```python
from build123d import *

# Parameters (mm, degrees)
F0_R     = 7.5
F0_R_2   = 6.5
F1_DEPTH = 2.5
F0_R_3   = 4
F2_DEPTH = 2
F0_R_4   = 3
F3_DEPTH = 2.5


with BuildPart() as f1:
    # F0 (on Front) → F1 (new body, symmetric)
    with BuildSketch(Plane.XZ):
        Circle(F0_R)
        Circle(F0_R_2, mode=Mode.SUBTRACT)
    extrude(amount=F1_DEPTH, both=True)

    # F0 (on Front) → F2 (join, symmetric)
    with BuildSketch(Plane.XZ):
        Circle(F0_R_2)
        Circle(F0_R_3, mode=Mode.SUBTRACT)
    extrude(amount=F2_DEPTH, both=True)

    # F0 (on Front) → F3 (join, symmetric)
    with BuildSketch(Plane.XZ):
        Circle(F0_R_3)
        Circle(F0_R_4, mode=Mode.SUBTRACT)
    extrude(amount=F3_DEPTH, both=True)


solid = f1.part
```
The model under review builds one solid part; all positions refer to its coordinate system, in mm. A direction names the side the tool comes from. Round coordinates to 2 decimals unless told otherwise and drop trailing zeros. Loops run counter-clockwise (first coordinate to the right, second up) from the corner with the lowest first, then second, coordinate; pieces in that order, holes last. Notation, with made-up numbers: (-36.5, 19.5) - (-10.5, 19.5) arc R21 cw to (-10.5, 42.5) - close; hole circle Ø2 at (42, -0.75). An arc over 180 degrees is marked (long way). Write each question's results on one line, items separated by ' | '. Start each with the question number.
Q1. Take a section at B-B on x = 0. Give the boundary of the cut face in (y, z), plus the area to 3 significant figures.
Q2. Wall thickness on line 1 along Z through (x, y) = (0, 2.3); line 2 along Z through (x, y) = (0, -1.25); line 3 along Y through (x, z) = (-2, 4): over which ranges is each line inside the solid? List them lowest first. Write a range as [from, to].
Q3. Take a section at A-A on z = 0. Give the boundary of the cut face in (x, y), plus the area to 3 significant figures.
Q4. Take a section at D-D on x = -5.75. Give the boundary of the cut face in (y, z), plus the area to 3 significant figures.
Q5. Take a section at C-C on y = -0.8. Give the boundary of the cut face in (x, z), plus the area to 3 significant figures.
Q6. Draft analysis for pull direction Z (two halves, no side actions). For faces 1 (the cylindrical face through (-5.158, -2.246, -3.955)), 2 (the cylindrical face through (-7.493, -0.035, 0.33)), 3 (the flat face through (1, -2.5, 3)), state which applies: pulls with the +Z half, pulls with the -Z half, needs draft (parallel to the pull), parting line crosses it, or undercut.
Q7. Tool access review of faces 4 (the flat face through (1, 2.5, 3)), 5 (the cylindrical face through (-5.158, 2.254, -3.955)), 6 (the flat face through (3, -2, 3)): name each direction out of +Z, -Z, +X, -X, +Y, -Y from which nothing blocks a thin tool from reaching the whole face with its end or side.
Q8. Insertion check: P1, Ø1.5, axis at x = 2.5, y = 1, coming from the -Z side; P2, Ø3, axis at x = -5.5, y = 1.5, coming from the +Z side; P3, Ø1, axis at x = 6, y = 1, coming from the -Z side. Each pin has a flat end and moves straight along its axis. Give the tip position at first contact, or say it passes through.
Data:
1) outline: (-2.5, -7.5) - (2.5, -7.5) - (2.5, -6.5) - (2, -6.5) - (2, -4) - (2.5, -4) - (2.5, -3) - (-2.5, -3) - (-2.5, -4) - (-2, -4) - (-2, -6.5) - (-2.5, -6.5) - close; (-2.5, 3) - (2.5, 3) - (2.5, 4) - (2, 4) - (2, 6.5) - (2.5, 6.5) - (2.5, 7.5) - (-2.5, 7.5) - (-2.5, 6.5) - (-2, 6.5) - (-2, 4) - (-2.5, 4) - close | area: 40.0 mm²
2) line 1: z = [-7.5, -6.5], [-4, -3], [3, 4], [6.5, 7.5] | line 2: z = [-7.5, -3], [3, 7.5] | line 3: y = [-2, 2]
3) outline: (-7.5, -2.5) - (-6.5, -2.5) - (-6.5, -2) - (-4, -2) - (-4, -2.5) - (-3, -2.5) - (-3, 2.5) - (-4, 2.5) - (-4, 2) - (-6.5, 2) - (-6.5, 2.5) - (-7.5, 2.5) - close; (3, -2.5) - (4, -2.5) - (4, -2) - (6.5, -2) - (6.5, -2.5) - (7.5, -2.5) - (7.5, 2.5) - (6.5, 2.5) - (6.5, 2) - (4, 2) - (4, 2.5) - (3, 2.5) - close | area: 40.0 mm²
4) outline: (-2.5, -4.82) - (2.5, -4.82) - (2.5, -3.03) - (2, -3.03) - (2, 3.03) - (2.5, 3.03) - (2.5, 4.82) - (-2.5, 4.82) - (-2.5, 3.03) - (-2, 3.03) - (-2, -3.03) - (-2.5, -3.03) - close | area: 42.1 mm²
5) outline: circle Ø15 at (0, 0); hole circle Ø6 at (0, 0) | area: 148 mm²
6) face 1: undercut | face 2: parting line crosses it | face 3: needs draft
7) face 4: +Z, -Z, +X, -X, +Y | face 5: +Y | face 6: -Y
8) P1: stops at z = -7.29 | P2: stops at z = 6.34 | P3: stops at z = -5.1
